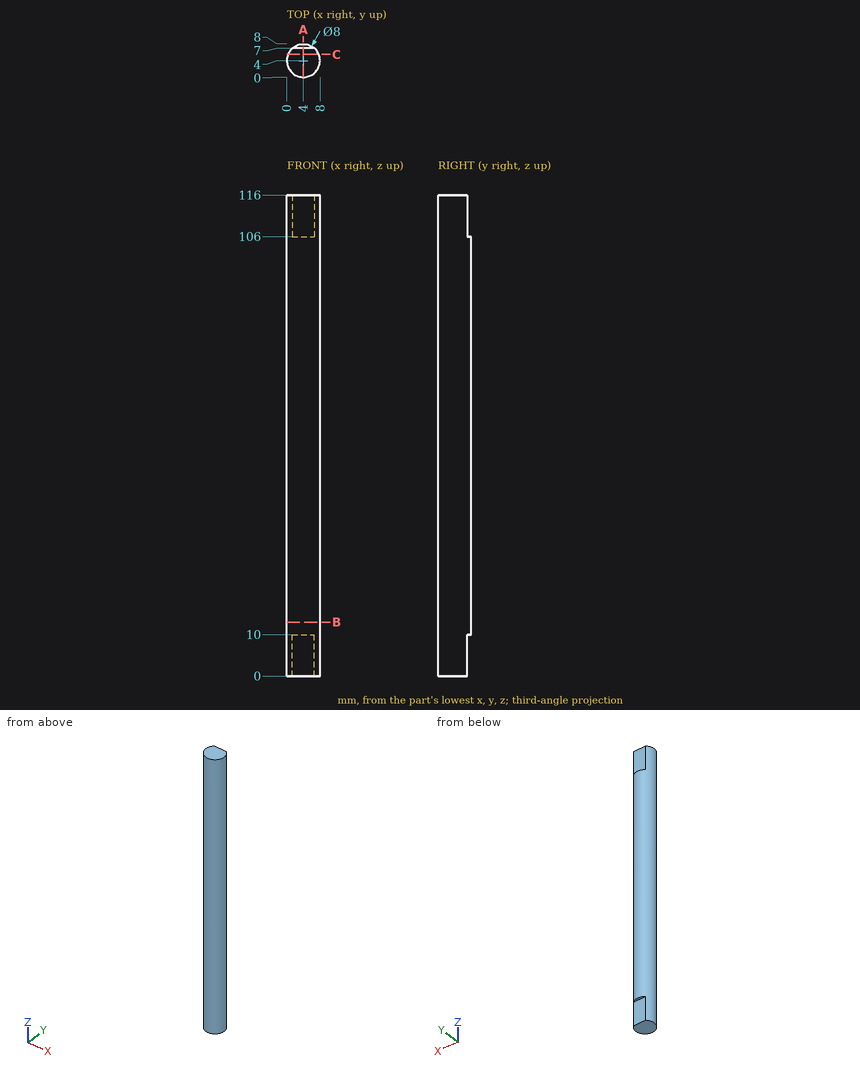
For this review, use the dimensioned drawing (mm, ordinates from the lowest corner) and the shaded views. Give positions to 0.01 mm unless a question says otherwise; leave off trailing zeros. Order: outer loops, then holes, each group sorted by start corner. A loop starts at its lowest first (then second) coordinate and runs counter-clockwise, first axis right, second up.
1) Insertion check: pin 1 (2.5 mm diameter, centred on x = 5, z = 3.5, fed in from +Y). The pin has a flat end and moves straight along its axis. Give the tip position at first contact, or say it passes through.
2) Wall thickness on line 1 (X direction, y = 3.75, z = 76); line 2 (X direction, y = 0.5, z = 93): over which ranges is each line inside the solid? List them lowest first.
3) Take a section at C-C (y = 5.5). Give the boundary of the cut face in (x, z), then the cut area to 3 significant figures.
4) Take a section at B-B (z = 13). Give the boundary of the cut face in (x, y).
5) Take a section at A-A (x = 4). Give the boundary of the cut face in (y, z), then the cut area to 3 significant figures.
Derived:
1. pin 1: stops at y = 7
2. line 1: x = 0.01 to 7.99
2. line 2: x = 2.06 to 5.94
3. outline: (0.29, 0) - (7.71, 0) - (7.71, 116) - (0.29, 116) - close
3. area: 860 mm2
4. outline: circle Ø8 at (4, 4)
5. outline: (0, 0) - (7, 0) - (7, 10) - (8, 10) - (8, 106) - (7, 106) - (7, 116) - (0, 116) - close
5. area: 908 mm2
